```python
from build123d import *

# Parameters (mm, degrees)
CYLINDER183_R     = 1.25
CYLINDER183_DEPTH = 10
CYLINDER182_R     = 1.25
CYLINDER182_DEPTH = 10
CYLINDER181_R     = 1.25
CYLINDER181_DEPTH = 10
CYLINDER180_R     = 1.25
CYLINDER180_DEPTH = 10
BOX092_W          = 135
BOX092_H          = 10
BOX092_DEPTH      = 15
FILLET049_R       = 3
BOX093_W          = 135
BOX093_H          = 10
BOX093_DEPTH      = 15


with BuildPart() as cylinder183:
    # Cylinder183 → Cylinder183 (new body)
    with BuildSketch(Plane(origin=(564, 0, 10), x_dir=(1, 0, 0), z_dir=(0, -1, 0))):
        Circle(CYLINDER183_R)
    extrude(amount=CYLINDER183_DEPTH)


with BuildPart() as cylinder182:
    # Cylinder182 → Cylinder182 (new body)
    with BuildSketch(Plane(origin=(546, 0, 10), x_dir=(1, 0, 0), z_dir=(0, -1, 0))):
        Circle(CYLINDER182_R)
    extrude(amount=CYLINDER182_DEPTH)


with BuildPart() as cylinder181:
    # Cylinder181 → Cylinder181 (new body)
    with BuildSketch(Plane(origin=(459, 0, 10), x_dir=(1, 0, 0), z_dir=(0, -1, 0))):
        Circle(CYLINDER181_R)
    extrude(amount=CYLINDER181_DEPTH)


with BuildPart() as fusion155:
    # Cylinder180 → Cylinder180 (new body)
    with BuildSketch(Plane(origin=(441, 0, 10), x_dir=(1, 0, 0), z_dir=(0, -1, 0))):
        Circle(CYLINDER180_R)
    extrude(amount=CYLINDER180_DEPTH)

    # Fusion155: union Cylinder183, Cylinder182, Cylinder181
    add(cylinder183.part)
    add(cylinder182.part)
    add(cylinder181.part)


with BuildPart() as fillet049:
    # Box092 → Box092 (new body)
    with BuildSketch(Plane(origin=(435, 0, 5), x_dir=(1, 0, 0), z_dir=(0, 0, 1))):
        with Locations((67.5, 5)):
            Rectangle(BOX092_W, BOX092_H)
    extrude(amount=BOX092_DEPTH)

    # Fillet049
    fillet049_edges = [fillet049.edges().sort_by_distance(p)[0] for p in [
        (502.5, 0, 20),
    ]]
    fillet(fillet049_edges, radius=FILLET049_R)


with BuildPart() as fenders_holes:
    # Box093 → Box093 (new body)
    with BuildSketch(Plane(origin=(435, -4, 5), x_dir=(1, 0, 0), z_dir=(0, 0, 1))):
        with Locations((67.5, 5)):
            Rectangle(BOX093_W, BOX093_H)
    extrude(amount=BOX093_DEPTH)

    # Cut112: cut Fillet049
    add(fillet049.part, mode=Mode.SUBTRACT)

    # Cut113: cut Fusion155
    add(fusion155.part, mode=Mode.SUBTRACT)


solid = fenders_holes.part
```
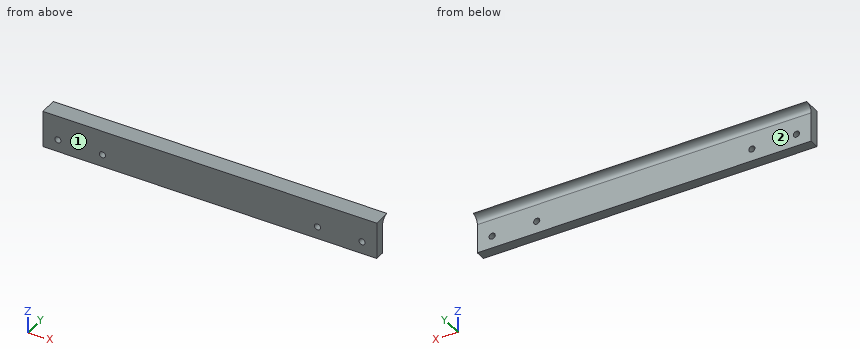
Build history of the part. All positions in model axes, mm. Face numbers are marked on the shaded views. A direction names the side the tool comes from. Round coordinates to 2 decimals unless told otherwise and drop trailing zeros. Loops run counter-clockwise (first coordinate to the right, second up) from the corner with the lowest first, then second, coordinate; pieces in that order, holes last.
Item 1: Pin check, flat tips, straight feed: P1, Ø2, axis at x = 459, z = 10, coming from the +Y side; P2, Ø2, axis at x = 468.5, z = 10.5, coming from the +Y side. Stop position of each tip, or through.
Item 2: Saw through at C-C (z = 18.5). List the corners of the cut face in (x, y).
Item 3: Saw through at B-B (z = 10). List the corners of the cut face in (x, y).
Item 4: Drill centre lines: line 1 along X through (y, z) = (-2.7, 10); line 2 along Z through (x, y) = (459, -1.2); line 3 along Y through (x, z) = (546.5, 8.5). Where is each one in solid material? Low to high.
Item 5: Saw through at A-A (x = 546). List the corners of the cut face in (y, z).
Item 6: Which spindle directions (+Z, -Z, +X, -X, +Y, -Y) get a long thin tool onto all of the face, cutting with end or side? Do the marked faces 1 and 2. Say none if no direction does.
Worked answers:
1. P1: passes through
1. P2: stops at y = 0
2. outline: (435, -4) - (570, -4) - (570, 0.4) - (435, 0.4) - close
3. outline: (435, -4) - (439.75, -4) - (439.75, 0) - (435, 0) - close; (442.25, -4) - (457.75, -4) - (457.75, 0) - (442.25, 0) - close; (460.25, -4) - (544.75, -4) - (544.75, 0) - (460.25, 0) - close; (547.25, -4) - (562.75, -4) - (562.75, 0) - (547.25, 0) - close; (565.25, -4) - (570, -4) - (570, 0) - (565.25, 0) - close
4. line 1: x = 435 to 439.75, 442.25 to 457.75, 460.25 to 544.75, 547.25 to 562.75, 565.25 to 570
4. line 2: z = 5 to 8.75, 11.25 to 20
4. line 3: y = -4 to 0
5. outline: (-4, 5) - (0, 5) - (0, 8.75) - (-4, 8.75) - close; (-4, 11.25) - (0, 11.25) - (0, 17) arc R3 cw to (3, 20) - (-4, 20) - close
6. face 1: +Z, -Z, +X, -X, -Y
6. face 2: -Z, +X, -X, +Y
